Autodesk Inventor part; units mm, degrees
ref_plane "YZ Plane" through (0, 0, 0) normal (1, 0, 0) x (0, 1, 0)
ref_plane "XZ Plane" through (0, 0, 0) normal (0, 1, 0) x (-1, 0, 0)
ref_plane "XY Plane" through (0, 0, 0) normal (0, 0, 1) x (1, 0, 0)
sketch "Sketch1" plane through (0, 0, 0) normal (0, 1, 0) x (-1, 0, 0)
  circle A0 centre (0, 0) radius 3.5
  circle A1 centre (0, -20) radius 3.5
  line L0 (3.5, 0) -> (3.5, -20)
  line L1 (-3.5, -20) -> (-3.5, 0)
  line L2 (0, 0) -> (0, -20) construction
  circle A2 centre (0, 0) radius 1.25
  circle A3 centre (0, -20) radius 1.25
  circle A4 centre (0, -20) radius 2.5
  circle A5 centre (0, 0) radius 2.5
  dimension "d0" = 7
  dimension "d1" = 2.5
  dimension "d2" = 20
  dimension "d5" = 5
  dimension "d6" = 5
extrude "Extrusion1" add sketch "Sketch1" along normal blind 3 contours A0 | L0 A1 L1 A0 | A1
extrude "Extrusion2" add sketch "Sketch1" along normal blind 1 contours A4 | A5
properties part number "Link_3DPrint"
Could you check a few things on this model? Use its own coordinates, in mm. A direction names the side the tool comes from. Coordinates: 2 decimals unless noted, no trailing zeros. Write each loop counter-clockwise with the first axis right and the second up, starting at its lowest first coordinate (ties: lowest second). Pieces come first, ordered by that corner, then holes. Notation, with made-up numbers: (59.5, 38.25) - (68.5, 38.25) arc R19 cw to (68.5, 75.25) - close; hole circle Ø9 at (61, 3). An arc over 180 degrees is marked (long way). Use a Markdown table: item, result.
Q1. Thinking about a two-plate mould opening in Z: for faces 3 (the flat face through (1, 1, -21)), 4 (the cylindrical face through (0.1, 1.5, 3.5)), 5 (the cylindrical face through (0.27, 0.49, -18.78)), 6 (the cylindrical face through (-0.1, 1.5, -23.5)), which applies, +Z half, -Z half, draft (parallel to the pull), parting line (faces both ways), or undercut?
Geometry check:
| item | result |
|---|---|
| face 3 | undercut |
| face 4 | +Z half |
| face 5 | undercut |
| face 6 | -Z half |
Q2. Imagine slicing it at B-B (y = 1.9). List the corners of the cut face in (x, z) for me, and give its area (3 significant figures).
Geometry check:
| item | result |
|---|---|
| outline | (-3.5, -20) arc R3.5 ccw to (3.5, -20) - (3.5, 0) arc R3.5 ccw to (-3.5, 0) - close; hole circle Ø5 at (0, -20); hole circle Ø5 at (0, 0) |
| area | 139 mm2 |
Q3. Imagine slicing it at C-C (z = -19.25). List the corners of the cut face in (x, y) for me.
Geometry check:
| item | result |
|---|---|
| outline | (-3.5, 0) - (-1, 0) - (-1, 1) - (-2.38, 1) - (-2.38, 3) - (-3.5, 3) - close; (1, 0) - (3.5, 0) - (3.5, 3) - (2.38, 3) - (2.38, 1) - (1, 1) - close |
Q4. Please list where these lines run through material, in increasing order: L1, parallel to Z at x = 0, y = 0.6; L2, parallel to Z at x = 0, y = 1.45; L3, parallel to X at y = 0.95, z = -1.
Geometry check:
| item | result |
|---|---|
| L1 | z = -23.5 to -21.25, -18.75 to -1.25, 1.25 to 3.5 |
| L2 | z = -23.5 to -22.5, -17.5 to -2.5, 2.5 to 3.5 |
| L3 | x = -3.5 to -0.75, 0.75 to 3.5 |
Q5. Which directions (+Z, -Z, +X, -X, +Y, -Y) give clear straight access to the entire face, cutting with the end or side of a thin tool? Please do faces 1 (the cylindrical face through (0.27, 0.49, 1.22)), 2 (the cylindrical face through (0.33, 1.99, -22.48)).
Geometry check:
| item | result |
|---|---|
| face 1 | +Y, -Y |
| face 2 | +Y |
Q6. Imagine slicing it at A-A (x = 0). List the corners of the cut face in (y, z) for me, and give its area (3 significant figures).
Geometry check:
| item | result |
|---|---|
| outline | (0, -23.5) - (3, -23.5) - (3, -22.5) - (1, -22.5) - (1, -21.25) - (0, -21.25) - close; (0, -18.75) - (1, -18.75) - (1, -17.5) - (3, -17.5) - (3, -2.5) - (1, -2.5) - (1, -1.25) - (0, -1.25) - close; (0, 1.25) - (1, 1.25) - (1, 2.5) - (3, 2.5) - (3, 3.5) - (0, 3.5) - close |
| area | 56.0 mm2 |
Q7. I'm going to push flat-ended pins straight in: pin 1 Ø4 at (x, z) = (0, -20) entering from +Y; pin 2 Ø1 at (x, y) = (-2, 1.5) entering from -Z. Where does each tip first touch, or does it pass through?
Geometry check:
| item | result |
|---|---|
| pin 1 | stops at y = 1 |
| pin 2 | stops at z = -23.16 |
Q8. Imagine slicing it at D-D (z = 1.75). List the corners of the cut face in (x, y) for me, and give its area (3 significant figures).
Geometry check:
| item | result |
|---|---|
| outline | (-3.03, 0) - (3.03, 0) - (3.03, 3) - (1.79, 3) - (1.79, 1) - (-1.79, 1) - (-1.79, 3) - (-3.03, 3) - close |
| area | 11.0 mm2 |
